Geometry check sheet. Reference: the model listing, model coordinates, mm. A direction names the side the tool comes from. Give positions to 0.01 mm unless a question says otherwise; leave off trailing zeros. Loops run counter-clockwise (first coordinate to the right, second up) from the corner with the lowest first, then second, coordinate; pieces in that order, holes last. Notation, with made-up numbers: (16.25, 82) -> (44.25, 82) arc R20 ccw to (44.25, 103) -> close; hole circle Ø11 at (80, -36.5). An arc over 180 degrees is marked (long way). Answer as a JSON object with one key per item and string values.
from build123d import *

# Parameters (mm, degrees)
SKETCH_1_W          = 198
SKETCH_1_H          = 98
EXTRUDE_1_DEPTH     = 42
SKETCH_2_R          = 1.5
CUT_EXTRUDE_1_DEPTH = 3
SKETCH_3_R          = 28.5
SKETCH_3_R_2        = 5
CUT_EXTRUDE_2_DEPTH = 2


with BuildPart() as part:
    # 草图1 → 凸台-拉伸1 (new body)
    with BuildSketch(Plane(origin=(0, 0, 0), x_dir=(1, 0, 0), z_dir=(0, 1, 0))):
        with Locations((99, -49)):
            Rectangle(SKETCH_1_W, SKETCH_1_H)
    extrude(amount=EXTRUDE_1_DEPTH)

    # 草图2 → 切除-拉伸1 (cut)
    with BuildSketch(Plane(origin=(0, 42, 0), x_dir=(1, 0, 0), z_dir=(0, 1, 0))):
        with Locations(Location((61, -10, 0), (0, 0, 270))):
            Circle(SKETCH_2_R)
        with Locations(Location((181, -10, 0), (0, 0, 270))):
            Circle(SKETCH_2_R)
        with Locations(Location((181, -90, 0), (0, 0, 270))):
            Circle(SKETCH_2_R)
        with Locations(Location((61, -90, 0), (0, 0, 270))):
            Circle(SKETCH_2_R)
    extrude(amount=-CUT_EXTRUDE_1_DEPTH, mode=Mode.SUBTRACT)

    # 草图3 → 切除-拉伸2 (cut)
    with BuildSketch(Plane.XZ):
        with Locations(Location((153, 35, 0), (0, 0, 270))):
            Circle(SKETCH_3_R)
        with Locations(Location((153, 35, 0), (0, 0, 270))):
            Circle(SKETCH_3_R_2, mode=Mode.SUBTRACT)
    extrude(amount=-CUT_EXTRUDE_2_DEPTH, mode=Mode.SUBTRACT)


solid = part.part
1) Draft check along X on faces 3 (the face through (198, 21, 50)), 4 (the face through (98, 0, 48)), 5 (the face through (0, 21, 50)), 6 (the face through (127.716, 0.986, 21.849)). Enter one of: pulls with the +X half, pulls with the -X half, needs draft (parallel to the pull), parting line crosses it, or undercut.
Geometry check:
{"face 3": "pulls with the +X half", "face 4": "needs draft", "face 5": "pulls with the -X half", "face 6": "undercut"}
2) Material ranges on line 1 along X through (y, z) = (40.05, 10); line 2 along X through (y, z) = (1.15, 35); line 3 along Z through (x, y) = (181, 40.55), recorded low to high. Write a range as from..to.
Geometry check:
{"line 1": "x = 0..59.5, 62.5..179.5, 182.5..198", "line 2": "x = 0..124.5, 148..158, 181.5..198", "line 3": "z = 0..8.5, 11.5..88.5, 91.5..98"}
3) Section check A-A on x = 153. Record the cut outline in (y, z).
Geometry check:
{"outline": "(0, 0) -> (42, 0) -> (42, 98) -> (0, 98) -> (0, 63.5) -> (2, 63.5) -> (2, 40) -> (0, 40) -> (0, 30) -> (2, 30) -> (2, 6.5) -> (0, 6.5) -> close"}
4) Tool access check on faces 1 (the face through (98, 21, 0)), 2 (the face through (153, 2, 29)). Record the directions out of +Z, -Z, +X, -X, +Y, -Y that give a thin tool (end or side, any length) a straight path to the whole face; none if there is none.
Geometry check:
{"face 1": "-Z, +X, -X, +Y, -Y", "face 2": "-Y"}
5) Depth check by flat-ended pin: P1, Ø2.5, axis at x = 181, z = 10, coming from the -Y side; P2, Ø1.5, axis at x = 60.5, z = 9.5, coming from the +Y side. Enter the tip coordinate at first touch or a pass-through.
Geometry check:
{"P1": "stops at y = 0", "P2": "stops at y = 39"}
